For this review, take the finished solid that the model builds, in its own axes (mm). A direction names the side the tool comes from. Round coordinates to 2 decimals unless told otherwise and drop trailing zeros. Write each loop counter-clockwise with the first axis right and the second up, starting at its lowest first coordinate (ties: lowest second). Pieces come first, ordered by that corner, then holes. Notation, with made-up numbers: M 32.25,-12.75 L 51.25,-12.75 A20 cw 51.25,23.25 Z; hole C 7,10.25 d11. An arc over 180 degrees is marked long. Answer in a Markdown table with one row per item.
```python
from build123d import *

# Parameters (mm, degrees)
F1_R     = 1.6
F2_DEPTH = 2.5
F3_W     = 7
F3_H     = 18.5
F4_DEPTH = 2.5
F5_R     = 1.6
F6_DEPTH = 2.5


with BuildPart() as f2:
    # F1 (on offset) → F2 (new body)
    with BuildSketch(Plane.XY.offset(16)):
        with BuildLine():
            ThreePointArc((48.0560038294, 18.8446410406), (49.5170345112, 20.1361157487), (50.0602513075, 22.0089299644))
            ThreePointArc((50.0602513075, 22.0089299644), (48.4330655233, 24.9657131681), (45.0644987857, 25.1732188883))
            ThreePointArc((45.0644987857, 25.1732188883), (43.3959623837, 20.5131774426), (48.0560038294, 18.8446410406))
        make_face()
        with Locations((46.5602513075, 22.0089299644)):
            Circle(F1_R, mode=Mode.SUBTRACT)
        with BuildLine():
            ThreePointArc((48.0560038294, 18.8446410406), (43.3959623837, 20.5131774426), (45.0644987857, 25.1732188883))
            Line((45.0644987857, 25.1732188883), (21.7843731319, 14.168753906))
            Line((21.7843731319, 14.168753906), (24.7758781756, 7.8401760584))
            Line((24.7758781756, 7.8401760584), (48.0560038294, 18.8446410406))
        make_face()
    extrude(amount=F2_DEPTH)

    # F3 (on face) → F4 (join)
    with BuildSketch(Plane(origin=(23.2801256538, 11.0044649822, 0), x_dir=(0.4273578634, -0.9040825497, 0), z_dir=(-0.9040825497, -0.4273578634, 0))):
        with Locations((0, 9.25)):
            Rectangle(F3_W, F3_H)
    extrude(amount=F4_DEPTH)

    # F5 (on Top) → F6 (join)
    with BuildSketch(Plane.XY):
        with BuildLine():
            ThreePointArc((1.4957525219, -3.1642889238), (2.9567832036, -1.8728142158), (3.5, 0))
            ThreePointArc((3.5, 0), (1.8728142158, 2.9567832036), (-1.4957525219, 3.1642889238))
            ThreePointArc((-1.4957525219, 3.1642889238), (-3.1642889238, -1.4957525219), (1.4957525219, -3.1642889238))
        make_face()
        Circle(F5_R, mode=Mode.SUBTRACT)
        with BuildLine():
            ThreePointArc((-1.4957525219, 3.1642889238), (1.8728142158, 2.9567832036), (3.5, 0))
            ThreePointArc((3.5, 0), (2.9567832036, -1.8728142158), (1.4957525219, -3.1642889238))
            Line((1.4957525219, -3.1642889238), (22.5156718015, 6.7717813999))
            Line((22.5156718015, 6.7717813999), (19.5241667578, 13.1003592476))
            Line((19.5241667578, 13.1003592476), (-1.4957525219, 3.1642889238))
        make_face()
    extrude(amount=F6_DEPTH)


solid = f2.part
```
Q1. Mouldability with a two-part tool opening along Y and no side actions: class faces 4 (the face through (-3.196, -1.426, 1.232)), 5 (the face through (-1.27, -0.97, 1.23)), 6 (the face through (44.96, 22.08, 17.23)), 7 (the face through (10, 5, 0)) as +Y half, -Y half, draft (parallel to the pull), parting line (faces both ways), or undercut.
Found:
| item | result |
|---|---|
| face 4 | parting line |
| face 5 | undercut |
| face 6 | undercut |
| face 7 | draft |
Q2. For probe 1 along Z at (x, y) = (26, 8.75); probe 2 along Y at (x, z) = (0, 1.85); probe 3 along X at (y, z) = (11.25, 14.25), list the stretches that pass through material, from the lowest coordinate up.
Found:
| item | result |
|---|---|
| probe 1 | 16 to 18.5 |
| probe 2 | -3.5 to -1.6, 1.6 to 3.87 |
| probe 3 | 20.4 to 23.16 |
Q3. Take a section at D-D (x = 11). State the section outline as (y, z) points, then the cut area to 3 significant figures.
Found:
| item | result |
|---|---|
| outline | M 1.33,0 L 9.07,0 L 9.07,2.5 L 1.33,2.5 Z |
| area | 19.4 mm² |
Q4. Take a section at B-B (x = 0). State the section outline as (y, z) points, then the cut area to 3 significant figures.
Found:
| item | result |
|---|---|
| outline | M -3.5,0 L -1.6,0 L -1.6,2.5 L -3.5,2.5 Z; M 1.6,0 L 3.87,0 L 3.87,2.5 L 1.6,2.5 Z |
| area | 10.4 mm² |
Q5. Machinability: for faces 1 (the face through (36, 17, 18.5)), 2 (the face through (21, 9.98, 10.61)), 3 (the face through (23.26, 11.05, 8.11)), which of the approach directions +Z, -Z, +X, -X, +Y, -Y give a long, thin tool a straight path to every point of the face, cutting with its end or side? Answer none if there is none.
Found:
| item | result |
|---|---|
| face 1 | +Z, +X, -X, +Y, -Y |
| face 2 | +Z, -X, -Y |
| face 3 | -Z, +X, +Y |
Q6. Insertion check: P1, Ø8.5, axis at x = 3.5, y = 2.5, coming from the +Z side; P2, Ø8, axis at y = 5, z = 8.5, coming from the -X side. Each pin has a flat end and moves straight along its axis. Give the tip position at first contact, or say it passes through.
Found:
| item | result |
|---|---|
| P1 | z = 2.5 |
| P2 | x = 21.46 |
Q7. Take a section at C-C (z = 6.25). State the section outline as (x, y) points.
Found:
| item | result |
|---|---|
| outline | M 19.52,13.1 L 22.52,6.77 L 24.78,7.84 L 21.78,14.17 Z |
Q8. Take a section at A-A (y = -0.75). State the section outline as (x, z) points, then the cut area to 3 significant figures.
Found:
| item | result |
|---|---|
| outline | M -3.42,0 L -1.41,0 L -1.41,2.5 L -3.42,2.5 Z; M 1.41,0 L 6.6,0 L 6.6,2.5 L 1.41,2.5 Z |
| area | 18.0 mm² |
